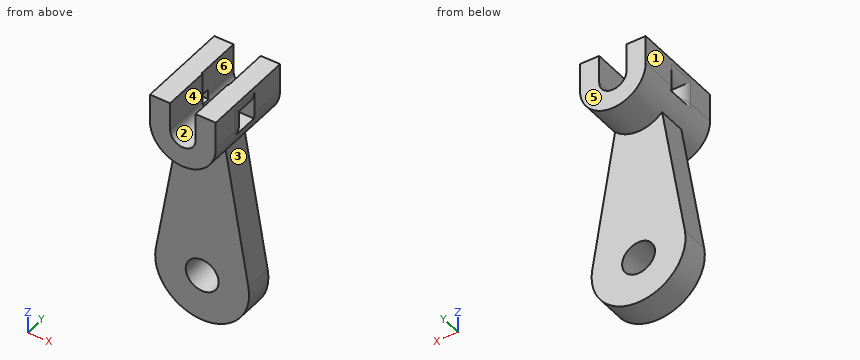
```python
from build123d import *

# Parameters (mm, degrees)
BOSS_EXTRUDE1_DEPTH     = 5
BOSS_EXTRUDE2_DEPTH     = 5
CUT_EXTRUDE1_DEPTH      = 12.694122455
CUT_EXTRUDE1_DEPTH_BACK = 12.694122455
SKETCH3_W               = 1
SKETCH3_H               = 1
FILLET1_R               = 2
BOSS_EXTRUDE3_START     = 3
SKETCH4_R               = 1.75
BOSS_EXTRUDE3_DEPTH     = 3


with BuildPart() as part:
    # Sketch1 → Boss-Extrude1 (new body)
    with BuildSketch(Plane(origin=(0, 0, 0), x_dir=(1, 0, 0), z_dir=(0, 1, 0))):
        with BuildLine():
            Line((-1.35, 0), (-1.35, -3))
            Line((-1.35, -3), (-3.5, -3))
            Line((-3.5, -3), (-3.5, 0))
            ThreePointArc((-3.5, 0), (0, 3.5), (3.5, 0))
            Line((3.5, 0), (3.5, -3))
            Line((3.5, -3), (1.35, -3))
            Line((1.35, -3), (1.35, 0))
            ThreePointArc((1.35, 0), (0, 1.35), (-1.35, 0))
        make_face()
    extrude(amount=BOSS_EXTRUDE1_DEPTH)

    # Sketch2 → Boss-Extrude2 (add)
    with BuildSketch(Plane(origin=(0, 5, 0), x_dir=(1, 0, 0), z_dir=(0, 1, 0))):
        with BuildLine():
            Line((-1.45, -2.9), (-1.45, 0))
            ThreePointArc((-1.45, 0), (0, 1.45), (1.45, 0))
            Line((1.45, 0), (1.45, -2.9))
            Line((1.45, -2.9), (1.45, -3))
            Line((1.45, -3), (3.5, -3))
            Line((3.5, -3), (3.5, 0))
            ThreePointArc((3.5, 0), (0, 3.5), (-3.5, 0))
            Line((-3.5, 0), (-3.5, -3))
            Line((-3.5, -3), (-1.45, -3))
            Line((-1.45, -3), (-1.45, -2.9))
        make_face()
    extrude(amount=BOSS_EXTRUDE2_DEPTH)

    # Sketch3 → Cut-Extrude1 (cut, two sides: drawn at the far end of the back side and taken through both)
    with BuildSketch(Plane(origin=(-1.45, 0, 0), x_dir=(0, 0, -1), z_dir=(1, 0, 0)).offset(-CUT_EXTRUDE1_DEPTH_BACK)):
        with Locations((0, 5.5)):
            Rectangle(SKETCH3_W, SKETCH3_H)
    extrude(amount=CUT_EXTRUDE1_DEPTH + CUT_EXTRUDE1_DEPTH_BACK, mode=Mode.SUBTRACT)

    # Fillet1
    fillet1_edges = [part.edges().sort_by_distance(p)[0] for p in [
        (3.5, 5.5, 0.5),
        (3.5, 5, 0.25),
        (-3.5, 5.5, 0.5),
        (3.491013868, 5, -0.250643519),
        (-3.5, 5, 0.25),
        (-3.491013868, 5, -0.250643519),
    ]]
    fillet(fillet1_edges, radius=FILLET1_R)

    # Sketch4 → Boss-Extrude3 (add)
    with BuildSketch(Plane.XZ.offset(-6).offset(BOSS_EXTRUDE3_START)):
        with BuildLine():
            Line((-4.930452649, -16.86895447), (-2.5, -2.449489743))
            ThreePointArc((-2.5, -2.449489743), (0, -3.5), (2.5, -2.449489743))
            Line((2.5, -2.449489743), (4.930452649, -16.86895447))
            ThreePointArc((4.930452649, -16.86895447), (0, -22.7), (-4.930452649, -16.86895447))
        make_face()
        with Locations(Location((0, -17.7, 0), (0, 0, 270))):
            Circle(SKETCH4_R, mode=Mode.SUBTRACT)
    extrude(amount=-BOSS_EXTRUDE3_DEPTH)


solid = part.part
```
Geometry: final body of the model. Coordinates: model frame, mm. Face numbers are marked on the shaded views. A direction names the side the tool comes from. Round coordinates to 2 decimals unless told otherwise and drop trailing zeros. Order: outer loops, then holes, each group sorted by start corner. A loop starts at its lowest first (then second) coordinate and runs counter-clockwise, first axis right, second up. Notation, with made-up numbers: (76.5, -36.5) - (128.5, -36.5) arc R16 ccw to (128.5, -12.5) - close; hole circle Ø3 at (26, 35.25). An arc over 180 degrees is marked (long way). Write item = value, one per line. Start each with the question number.
Q1. Cut plane B-B on y = 8. Return the cut outline in (x, z).
Q2. Cut plane A-A on z = -17.7. Return the cut outline in (x, y), and give its area (3 significant figures).
Q3. Cut plane C-C on x = 0. Return the cut outline in (y, z), and give its area (3 significant figures).
Q4. Pull-direction query (Z, two-part tool) for the marked faces 1, 2 and 3; classes: +Z half, -Z half, draft (parallel to the pull), parting line (faces both ways), or undercut.
Q5. Ray query, line 1 (X direction, y = 3.7, z = -17.7); line 2 (Y direction, x = -2, z = -18.5); line 3 (X direction, y = 2.75, z = -0.5). Return the intervals inside material, ascending. Write a range as from..to.
Q6. Pin query (flat end, axial travel): pin 1 (2 mm diameter, centred on x = 1, y = 7.5, fed in from -Z); pin 2 (2 mm diameter, centred on x = 0, z = -17.7, fed in from -Y); pin 3 (5 mm diameter, centred on x = 1.5, z = -9.5, fed in from -Y); pin 4 (6 mm diameter, centred on y = 4, z = -12, fed in from -X). Return the tip coordinate at first contact, or that it passes through.
Q7. Access query for the marked faces 4, 5 and 6. Directions: +Z, -Z, +X, -X, +Y, -Y. A direction counts if a zero-diameter tool reaches every point of the face in a straight line with its end or side. Return the directions, or none.
Q8. Cut plane D-D on y = 1.5. Return the cut outline in (x, z), and give its area (3 significant figures).
Outcome:
q1.outline = (-3.5, 0) arc R3.5 ccw to (3.5, 0) - (3.5, 3) - (1.45, 3) - (1.45, 0) arc R1.45 cw to (-1.45, 0) - (-1.45, 3) - (-3.5, 3) - close
q2.outline = (-5, 3) - (-1.75, 3) - (-1.75, 6) - (-5, 6) - close; (1.75, 3) - (5, 3) - (5, 6) - (1.75, 6) - close
q2.area = 19.5 mm^2
q3.outline = (0, -3.5) - (3, -3.5) - (3, -15.95) - (6, -15.95) - (6, -3.5) - (10, -3.5) - (10, -1.45) - (5, -1.45) - (5, -1.35) - (0, -1.35) - close; (3, -22.7) - (6, -22.7) - (6, -19.45) - (3, -19.45) - close
q3.area = 68.1 mm^2
q4.face_1 = draft
q4.face_2 = +Z half
q4.face_3 = undercut
q5.line_1 = -5..-1.75, 1.75..5
q5.line_2 = 3..6
q5.line_3 = -3.46..-1.25, 1.25..3.46
q6.pin_1 = -3.5
q6.pin_2 = through
q6.pin_3 = 3
q6.pin_4 = -4.62
q7.face_4 = +Z, +Y, -Y
q7.face_5 = +Z, -Z, +X, -X, +Y
q7.face_6 = +Z, +Y
q8.outline = (-3.5, 0) arc R3.5 ccw to (3.5, 0) - (3.5, 3) - (1.35, 3) - (1.35, 0) arc R1.35 cw to (-1.35, 0) - (-1.35, 3) - (-3.5, 3) - close
q8.area = 29.3 mm^2
